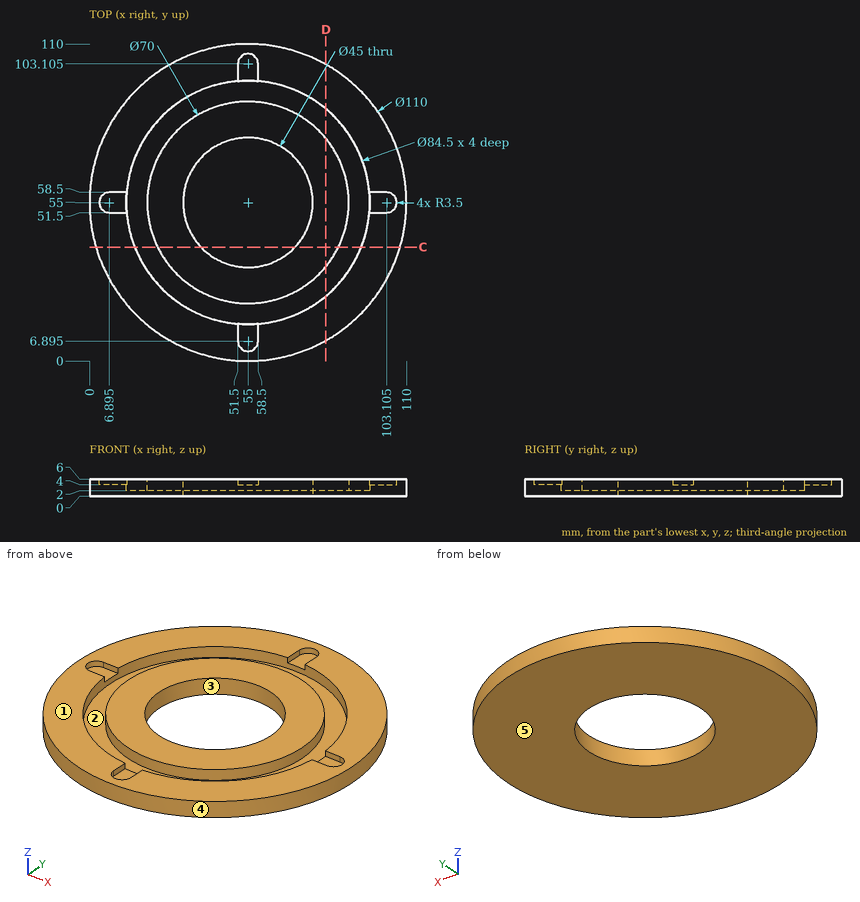
Part print with two shaded views. Sizes in mm from the minimum x, y, z corner. A direction names the side the tool comes from. Round coordinates to 2 decimals unless told otherwise and drop trailing zeros. Write each loop counter-clockwise with the first axis right and the second up, starting at its lowest first coordinate (ties: lowest second). Pieces come first, ordered by that corner, then holes. Notation, with made-up numbers: M 87.5,1 L 106.5,1 A19 ccw 106.5,7 Z; hole C 74.25,68 d7. An arc over 180 degrees is marked long. Put each result on its own line as item: value. Start each with the question number.
1) Pull direction X, two halves, no side cores. Call the marked faces 3, 4 and 5: pulls with the +X half, pulls with the -X half, needs draft (parallel to the pull), parting line crosses it, or undercut.
2) 3-axis set-ups, long thin cutter, end or side, ignore diameter. For the marked faces 1 and 2: which of +Z, -Z, +X, -X, +Y, -Y reach the whole face in a straight line?
3) Saw through at D-D, the plane x = 82. Write the cut outline in (y, z), and give its area (3 significant figures).
4) Drill centre lines: probe 1 along Y at (x, z) = (55, 4.1) (1 decimal); probe 2 along Y at (x, z) = (55, 3.4); probe 3 along X at (y, z) = (49, 2.35) (1 decimal). Where is each one in solid material? Low to high. Write a range as [from, to].
5) Pin check, flat tips, straight feed: pin 1 Ø3 at (x, y) = (39.5, 89.5) entering from +Z; pin 2 Ø0.6 at (x, z) = (99.5, 5) entering from -Y; pin 3 Ø1 at (x, z) = (22.5, 1.5) entering from +Y; pin 4 Ø5.5 at (x, y) = (103.5, 53.5) entering from +Z. Stop position of each tip, or through.
6) Saw through at C-C, the plane y = 39.5. Write the cut outline in (x, z).
Resolved:
1. face 3: undercut
1. face 4: parting line crosses it
1. face 5: needs draft
2. face 1: +Z, +X, -X, +Y, -Y
2. face 2: +Z
3. outline: M 7.08,0 L 102.92,0 L 102.92,6 L 87.5,6 L 87.5,2 L 77.27,2 L 77.27,6 L 32.73,6 L 32.73,2 L 22.5,2 L 22.5,6 L 7.08,6 Z
3. area: 493 mm²
4. probe 1: [0, 3.4], [20, 32.5], [77.5, 90], [106.6, 110]
4. probe 2: [0, 12.75], [20, 32.5], [77.5, 90], [97.25, 110]
4. probe 3: [0.3, 13.2], [20.5, 33.3], [76.7, 89.5], [96.8, 109.7]
5. pin 1: z = 2
5. pin 2: y = 22.27
5. pin 3: y = 99.73
5. pin 4: z = 6
6. outline: M 2.23,0 L 38.69,0 L 38.69,6 L 23.62,6 L 23.62,2 L 15.7,2 L 15.7,6 L 2.23,6 Z; M 71.31,0 L 107.77,0 L 107.77,6 L 94.3,6 L 94.3,2 L 86.38,2 L 86.38,6 L 71.31,6 Z
